Geometry check sheet. Reference: the model listing, model coordinates, mm. A direction names the side the tool comes from. Round coordinates to 2 decimals unless told otherwise and drop trailing zeros. Write each loop counter-clockwise with the first axis right and the second up, starting at its lowest first coordinate (ties: lowest second). Pieces come first, ordered by that corner, then holes. Notation, with made-up numbers: M -15.75,-31.75 L 18.25,-31.75 A19 ccw 18.25,-26.75 Z; hole C -16,31.25 d8. An arc over 180 degrees is marked long. Use a Markdown table: item, result.
```python
from build123d import *

# Parameters (mm, degrees)
F0_W     = 76.2
F0_H     = 152.4
F1_DEPTH = 38.1
F3_DEPTH = 76.201
F5_DEPTH = 76.201
F7_DEPTH = 76.201
F8_DEPTH = 76.201
F9_DEPTH = 73.026


with BuildPart() as f1:
    # F0 (on Top) → F1 (new body, symmetric)
    with BuildSketch(Plane.XY):
        Rectangle(F0_W, F0_H)
    extrude(amount=F1_DEPTH, both=True)

    # F2 (on face) → F3 (cut, through all)
    with BuildSketch(Plane.XY.offset(38.1)):
        Polygon((-9.525, 25.4), (-9.525, -6.35), (9.525, -6.35), (9.525, 25.4), (4.7625, 25.4), (4.7625, 6.35), (-4.7625, 6.35), (-4.7625, 25.4), align=None)
    extrude(amount=-F3_DEPTH, mode=Mode.SUBTRACT)

    # F4 (on face) → F5 (cut, through all)
    with BuildSketch(Plane(origin=(-38.1, 0, 0), x_dir=(0, -1, 0), z_dir=(-1, 0, 0))):
        Polygon((25.4, 9.525), (-6.35, 9.525), (-6.35, -9.525), (25.4, -9.525), (25.4, -4.7625), (6.35, -4.7625), (6.35, 4.7625), (25.4, 4.7625), align=None)
    extrude(amount=-F5_DEPTH, mode=Mode.SUBTRACT)

    # F6 (on face) → F7 (cut, through all)
    with BuildSketch(Plane.XY.offset(38.1)):
        with BuildLine():
            ThreePointArc((9.525, -18.653125), (8.711306, -16.688694), (6.746875, -15.875))
            ThreePointArc((6.746875, -15.875), (4.782444, -20.617556), (9.525, -18.653125))
        make_face()
        with BuildLine():
            ThreePointArc((22.621875, -15.875), (20.657444, -20.617556), (25.4, -18.653125))
            ThreePointArc((25.4, -18.653125), (24.586306, -16.688694), (22.621875, -15.875))
        make_face()
        with BuildLine():
            ThreePointArc((21.997912, -37.697932), (21.123243, -35.674362), (19.05, -34.925))
            ThreePointArc((19.05, -34.925), (17.316332, -39.721502), (21.997912, -37.697932))
        make_face()
        with BuildLine():
            ThreePointArc((10.995796, -37.376299), (10.599886, -35.946954), (9.525, -34.925))
            ThreePointArc((9.525, -34.925), (5.835455, -38.805645), (10.995796, -37.376299))
        make_face()
        with BuildLine():
            ThreePointArc((-5.702395, -37.499304), (-6.928701, -35.194996), (-9.525, -34.925))
            ThreePointArc((-9.525, -34.925), (-10.032339, -39.803612), (-5.702395, -37.499304))
        make_face()
        with BuildLine():
            ThreePointArc((-16.36457, -37.701578), (-17.14576, -35.770198), (-19.05, -34.925))
            ThreePointArc((-19.05, -34.925), (-21.13963, -39.632958), (-16.36457, -37.701578))
        make_face()
        with BuildLine():
            ThreePointArc((-6.746875, -15.875), (-8.711306, -16.688694), (-9.525, -18.653125))
            ThreePointArc((-9.525, -18.653125), (-6.746875, -21.43125), (-3.96875, -18.653125))
            ThreePointArc((-3.96875, -18.653125), (-4.782444, -16.688694), (-6.746875, -15.875))
        make_face()
        with BuildLine():
            ThreePointArc((-22.621875, -15.875), (-24.586306, -16.688694), (-25.4, -18.653125))
            ThreePointArc((-25.4, -18.653125), (-22.621875, -21.43125), (-19.84375, -18.653125))
            ThreePointArc((-19.84375, -18.653125), (-20.657444, -16.688694), (-22.621875, -15.875))
        make_face()
        with BuildLine():
            ThreePointArc((-22.621875, -66.675), (-20.657444, -65.861306), (-19.84375, -63.896875))
            ThreePointArc((-19.84375, -63.896875), (-22.621875, -61.11875), (-25.4, -63.896875))
            ThreePointArc((-25.4, -63.896875), (-24.586306, -65.861306), (-22.621875, -66.675))
        make_face()
        with BuildLine():
            ThreePointArc((25.4, -63.896875), (20.657444, -61.932444), (22.621875, -66.675))
            ThreePointArc((22.621875, -66.675), (24.586306, -65.861306), (25.4, -63.896875))
        make_face()
    extrude(amount=-F7_DEPTH, mode=Mode.SUBTRACT)

    # F4 (on face) → F8 (cut, through all)
    with BuildSketch(Plane(origin=(-38.1, 0, 0), x_dir=(0, -1, 0), z_dir=(-1, 0, 0))):
        Polygon((-76.2, 34.925), (-6.35, 34.925), (-6.35, 19.05), (34.925, 19.05), (34.925, 4.7625), (76.2, 4.7625), (76.2, 38.1), (-76.2, 38.1), align=None)
        Polygon((-6.35, -34.925), (-76.2, -34.925), (-76.2, -38.1), (76.2, -38.1), (76.2, -4.7625), (34.925, -4.7625), (34.925, -19.05), (-6.35, -19.05), align=None)
    extrude(amount=-F8_DEPTH, mode=Mode.SUBTRACT)

    # F2 (on face) → F9 (cut, through all)
    with BuildSketch(Plane.XY.offset(38.1)):
        Polygon((-19.05, -34.925), (-19.05, -15.875), (-25.4, -15.875), (-25.4, -66.675), (25.4, -66.675), (25.4, -15.875), (19.05, -15.875), (19.05, -34.925), (9.525, -34.925), (9.525, -15.875), (-9.525, -15.875), (-9.525, -34.925), align=None)
    extrude(amount=-F9_DEPTH, mode=Mode.SUBTRACT)


solid = f1.part
```
Item 1: Mould release check, pull along Y, two halves, no side actions. Record for faces 1 (the face through (0, -15.875, 14)), 2 (the face through (-9, -69, 4.762)), 3 (the face through (9.525, 13, 0)): +Y half, -Y half, draft (parallel to the pull), parting line (faces both ways), or undercut.
Outcome:
| item | result |
|---|---|
| face 1 | -Y half |
| face 2 | draft |
| face 3 | undercut |
Item 2: Cross-section at A-A, the plane x = 15. Count the separate pieces of the cut face and the enclosed holes in it, and give its area (3 significant figures).
Outcome:
| item | result |
|---|---|
| separate pieces | 2 |
| enclosed holes | 1 |
| area | 6,120 mm2 |
Item 3: Material ranges on line 1 along Y through (x, z) = (1, -2.5) (3 decimals); line 2 along Y through (x, z) = (-5.5, 1.5) (3 decimals); line 3 along X through (y, z) = (18, 12.5) (1 decimal), recorded low to high. Write a range as from..to.
Outcome:
| item | result |
|---|---|
| line 1 | y = -76.2..-66.675, -15.875..-6.35, 6.35..76.2 |
| line 2 | y = -76.2..-66.675, -15.875..-6.35, 25.4..76.2 |
| line 3 | x = -38.1..-9.5, -4.8..4.8, 9.5..38.1 |
Item 4: Go/stop test with flat-tipped pins: pin 1 (1.5 mm diameter, centred on x = 29.5, z = 13.5, fed in from -Y) (3 decimals); pin 2 (5 mm diameter, centred on x = -22, z = -27, fed in from -Y); pin 3 (1 mm diameter, centred on x = -0.5, y = -11, fed in from +Z). Record where each tip stops, or that it passes through.
Outcome:
| item | result |
|---|---|
| pin 1 | stops at y = -34.925 |
| pin 2 | stops at y = 6.35 |
| pin 3 | stops at z = 19.05 |
Item 5: Cross-section at B-B, the plane y = 22. Record the cut outline in (x, z) (1 decimal), and give its area (3 significant figures).
Outcome:
| item | result |
|---|---|
| outline | M -38.1,-34.9 L -9.5,-34.9 L -9.5,34.9 L -38.1,34.9 Z; M -4.8,-34.9 L 4.8,-34.9 L 4.8,34.9 L -4.8,34.9 Z; M 9.5,-34.9 L 38.1,-34.9 L 38.1,34.9 L 9.5,34.9 Z |
| area | 4,660 mm2 |
Item 6: Access from +Z, -Z, +X, -X, +Y, -Y to the whole of each face (thin tool, end or side, straight path). Record for faces 4 (the face through (-22, -15.875, -14)), 5 (the face through (-32, -25.4, -7)), 6 (the face through (0, -66.675, 0)).
Outcome:
| item | result |
|---|---|
| face 4 | +Z, -Z, -Y |
| face 5 | +X, -X |
| face 6 | +Z, -Z |
